The listing builds one solid part. Answer for the finished solid, in the listing's coordinates (mm). A direction names the side the tool comes from. Coordinates: 2 decimals unless noted, no trailing zeros. Order: outer loops, then holes, each group sorted by start corner. A loop starts at its lowest first (then second) coordinate and runs counter-clockwise, first axis right, second up. Notation, with made-up numbers: (54, 8) -> (106, 8) arc R18 cw to (106, 24) -> close; hole circle Ø8 at (82, 58). An arc over 180 degrees is marked (long way). Return JSON: item names as keys, results as strings.
```python
from build123d import *

# Parameters (mm, degrees)
AUFSATZ_LINEAR_AUSTRAGEN1_DEPTH      = 20
SKIZZE2_W                            = 34
SKIZZE2_H                            = 43.5
SCHNITT_LINEAR_AUSTRAGEN1_DEPTH      = 105.522724802
SCHNITT_LINEAR_AUSTRAGEN2_DEPTH      = 105.522724802
SCHNITT_LINEAR_AUSTRAGEN2_DEPTH_BACK = 105.522724802
SKIZZE3_R                            = 5


with BuildPart() as part:
    # Skizze1 → Aufsatz-Linear austragen1 (new, symmetric)
    with BuildSketch(Plane(origin=(0, 0, 0), x_dir=(0, 0, -1), z_dir=(1, 0, 0))):
        Polygon((-25, 23.5), (10, 23.5), (10, 26.5), (-25, 26.5), (-25, 70), (-35, 70), (-35, 40), (-65, 40), (-65, 70), (-75, 70), (-75, -26.5), (10, -26.5), (10, -23.5), (-25, -23.5), align=None)
    extrude(amount=AUFSATZ_LINEAR_AUSTRAGEN1_DEPTH, both=True)

    # Skizze2 → Schnitt-Linear austragen1 (cut, through all)
    with BuildSketch(Plane.XY):
        with Locations((0, 48.25)):
            Rectangle(SKIZZE2_W, SKIZZE2_H)
    extrude(amount=SCHNITT_LINEAR_AUSTRAGEN1_DEPTH, mode=Mode.SUBTRACT)

    # Skizze3 → Schnitt-Linear austragen2 (cut, two sides: drawn at the far end of the back side and taken through both)
    with BuildSketch(Plane(origin=(0, 0, 0), x_dir=(1, 0, 0), z_dir=(0, 1, 0)).offset(-SCHNITT_LINEAR_AUSTRAGEN2_DEPTH_BACK)):
        with Locations(Location((0, 0, 0), (0, 0, 270))):
            Circle(SKIZZE3_R)
    extrude(amount=SCHNITT_LINEAR_AUSTRAGEN2_DEPTH + SCHNITT_LINEAR_AUSTRAGEN2_DEPTH_BACK, mode=Mode.SUBTRACT)


solid = part.part
```
Item 1: The part is cut by section B-B on y = 49. Determine the outline of the cut face in (x, z).
Answer list:
{"outline": "(-20, 25) -> (-17, 25) -> (-17, 35) -> (-20, 35) -> close; (-20, 65) -> (-17, 65) -> (-17, 75) -> (-20, 75) -> close; (17, 25) -> (20, 25) -> (20, 35) -> (17, 35) -> close; (17, 65) -> (20, 65) -> (20, 75) -> (17, 75) -> close"}
Item 2: The part is cut by section D-D on x = -12. Determine the outline of the cut face in (y, z).
Answer list:
{"outline": "(-26.5, -10) -> (-23.5, -10) -> (-23.5, 25) -> (23.5, 25) -> (23.5, -10) -> (26.5, -10) -> (26.5, 75) -> (-26.5, 75) -> close"}
Item 3: The part is cut by section C-C on x = 0. Determine the outline of the cut face in (y, z).
Answer list:
{"outline": "(-26.5, -10) -> (-23.5, -10) -> (-23.5, -5) -> (-26.5, -5) -> close; (-26.5, 5) -> (-23.5, 5) -> (-23.5, 25) -> (23.5, 25) -> (23.5, 5) -> (26.5, 5) -> (26.5, 75) -> (-26.5, 75) -> close; (23.5, -10) -> (26.5, -10) -> (26.5, -5) -> (23.5, -5) -> close"}
Item 4: The part is cut by section A-A on z = 0. Determine the outline of the cut face in (x, y), plus the area to 3 significant figures.
Answer list:
{"outline": "(-20, -26.5) -> (-5, -26.5) -> (-5, -23.5) -> (-20, -23.5) -> close; (-20, 23.5) -> (-5, 23.5) -> (-5, 26.5) -> (-20, 26.5) -> close; (5, -26.5) -> (20, -26.5) -> (20, -23.5) -> (5, -23.5) -> close; (5, 23.5) -> (20, 23.5) -> (20, 26.5) -> (5, 26.5) -> close", "area": "180 mm2"}
Item 5: Which of the six approach directions +Z, -Z, +X, -X, +Y, -Y give full straight-line access (tool end or side, diameter ignored) to faces 5 (the flat face through (0, 0, 25)), 6 (the flat face through (20, 12, 52)), 7 (the flat face through (19, 55, 65)), 8 (the flat face through (17, 38, 50)), 9 (the flat face through (19, 70, 30))?
Answer list:
{"face 5": "-Z, +X, -X", "face 6": "+Z, -Z, +X, +Y, -Y", "face 7": "+X, -X, +Y", "face 8": "+Z, -Z, +Y", "face 9": "+Z, -Z, +X, -X, +Y"}
Item 6: Flat-ended cylindrical pins translate along their axes: pin 1 (2.5 mm diameter, centred on x = 18, y = 59.5, fed in from -Z); pin 2 (13 mm diameter, centred on x = 0, z = 0, fed in from +Y); pin 3 (0.9 mm diameter, centred on x = 18, z = 56.5, fed in from +Y). Find the tip coordinate at first contact, or state that the pin passes through.
Answer list:
{"pin 1": "z = 25", "pin 2": "y = 26.5", "pin 3": "y = 40"}
Item 7: Find the intervals of material crossed by probe 1 along Y at (x, z) = (-9, 23); probe 2 along Z at (x, y) = (0, 24); probe 3 along X at (y, z) = (28.5, 38), in increasing order.
Answer list:
{"probe 1": "-26.5 to -23.5, 23.5 to 26.5", "probe 2": "-10 to -5, 5 to 75", "probe 3": "-20 to -17, 17 to 20"}
Item 8: Determine the mould class of faces 1 (the flat face through (19, 40, 50)), 2 (the flat face through (-20, 12, 52)), 3 (the cylindrical face through (-4.88, -25.02, -1.08)), 4 (the flat face through (19, 48, 25)) for opening direction Z: pulls with the +Z half, pulls with the -Z half, needs draft (parallel to the pull), parting line crosses it, or undercut.
Answer list:
{"face 1": "undercut", "face 2": "needs draft", "face 3": "undercut", "face 4": "pulls with the -Z half"}
